Here's the drawing with two shaded views (mm, measured from the low corner). I have some questions. Round coordinates to 2 decimals unless told otherwise and drop trailing zeros. Order: outer loops, then holes, each group sorted by start corner. A loop starts at its lowest first (then second) coordinate and runs counter-clockwise, first axis right, second up. Notation, with made-up numbers: (29.5, 59) -> (65.5, 59) arc R21 cw to (65.5, 66) -> close; hole circle Ø11 at (21, -38). An arc over 180 degrees is marked (long way). Answer in a Markdown table with one row per item.
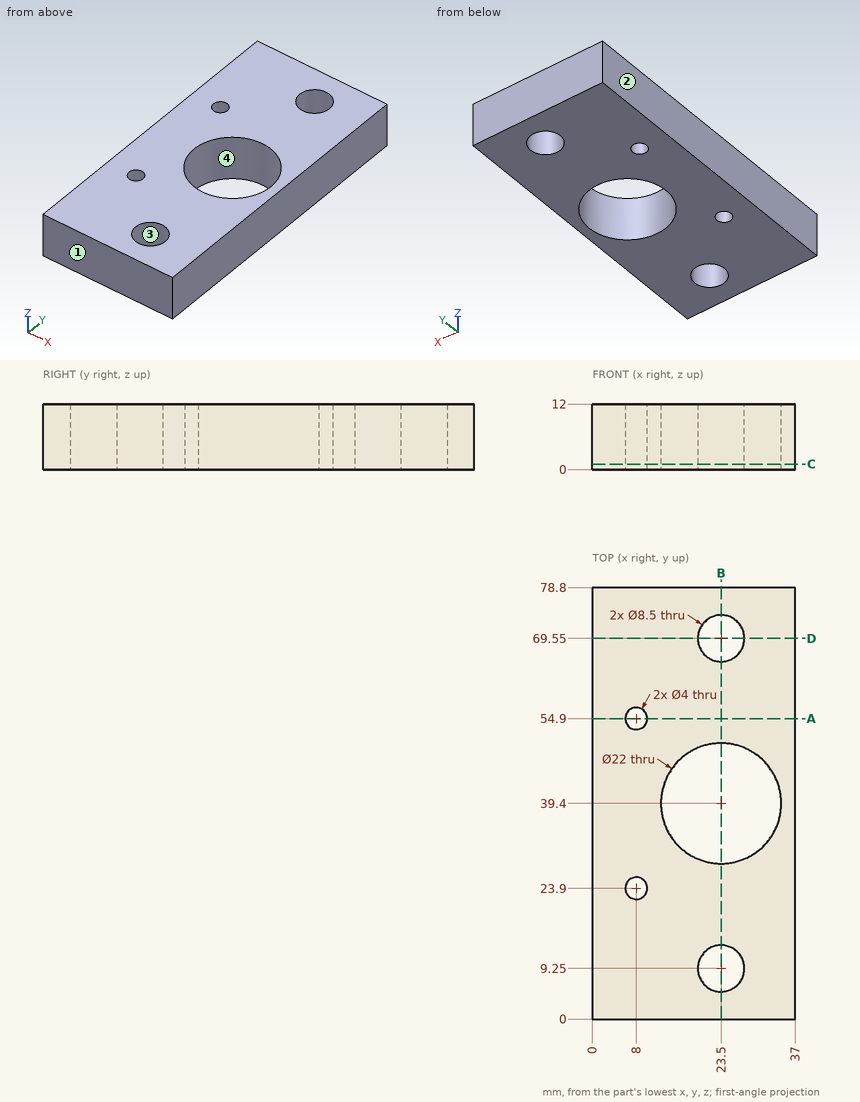
1. Suppose I cut it at C-C on z = 1. Write out the boundary of the cut face in (x, y), then the cut area to 3 significant figures.
Numbers:
| item | result |
|---|---|
| outline | (0, 0) -> (37, 0) -> (37, 78.8) -> (0, 78.8) -> close; hole circle Ø4 at (8, 23.9); hole circle Ø4 at (8, 54.9); hole circle Ø22 at (23.5, 39.4); hole circle Ø8.5 at (23.5, 9.25); hole circle Ø8.5 at (23.5, 69.55) |
| area | 2,400 mm2 |
2. Please list where these lines run through material, in increasing order: line 1 along Y through (x, z) = (23.5, 4.5); line 2 along Y through (x, z) = (8, 5.5); line 3 along Y through (x, z) = (20, 6.5).
Numbers:
| item | result |
|---|---|
| line 1 | y = 0 to 5, 13.5 to 28.4, 50.4 to 65.3, 73.8 to 78.8 |
| line 2 | y = 0 to 21.9, 25.9 to 52.9, 56.9 to 78.8 |
| line 3 | y = 0 to 6.84, 11.66 to 28.97, 49.83 to 67.14, 71.96 to 78.8 |
3. Suppose I cut it at B-B on x = 23.5. Write out the boundary of the cut face in (y, z).
Numbers:
| item | result |
|---|---|
| outline | (0, 0) -> (5, 0) -> (5, 12) -> (0, 12) -> close; (13.5, 0) -> (28.4, 0) -> (28.4, 12) -> (13.5, 12) -> close; (50.4, 0) -> (65.3, 0) -> (65.3, 12) -> (50.4, 12) -> close; (73.8, 0) -> (78.8, 0) -> (78.8, 12) -> (73.8, 12) -> close |
4. We'd pull the mould along X, two halves only. Please class the marked faces 1, 2, 3 and 4: released by +X, released by -X, zero draft, split by the parting line, or undercut.
Numbers:
| item | result |
|---|---|
| face 1 | zero draft |
| face 2 | released by -X |
| face 3 | undercut |
| face 4 | undercut |
5. Suppose I cut it at A-A on y = 54.9. Write out the boundary of the cut face in (x, z).
Numbers:
| item | result |
|---|---|
| outline | (0, 0) -> (6, 0) -> (6, 12) -> (0, 12) -> close; (10, 0) -> (37, 0) -> (37, 12) -> (10, 12) -> close |
6. Suppose I cut it at D-D on y = 69.55. Write out the boundary of the cut face in (x, z).
Numbers:
| item | result |
|---|---|
| outline | (0, 0) -> (19.25, 0) -> (19.25, 12) -> (0, 12) -> close; (27.75, 0) -> (37, 0) -> (37, 12) -> (27.75, 12) -> close |
